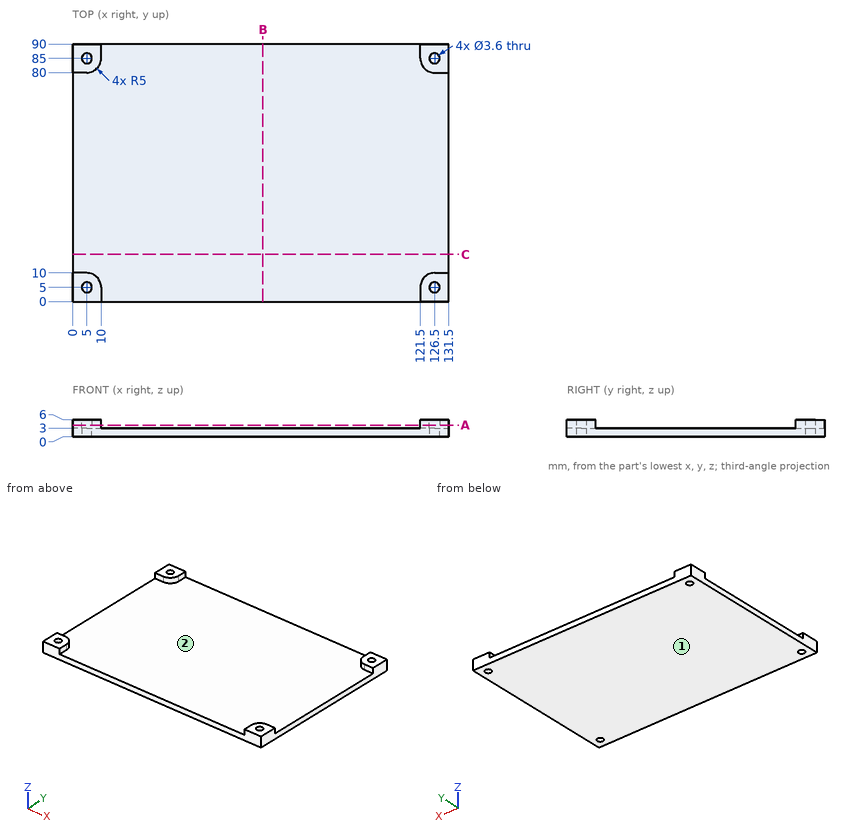
Answer from the drawing. Dimensions are ordinates in mm from the lowest x, y and z of the part. Coordinates: 2 decimals unless noted, no trailing zeros. Loops run counter-clockwise (first coordinate to the right, second up) from the corner with the lowest first, then second, coordinate; pieces in that order, holes last. Notation, with made-up numbers: (9.5, 62) -> (55.5, 62) arc R11 ccw to (55.5, 80) -> close; hole circle Ø7 at (41.5, 7). An arc over 180 degrees is marked (long way). Return JSON: item names as keys, results as strings.
Item 1: A flat-ended cylindrical pin translates along its axis: P1, Ø2.5, axis at x = 128, z = 4.5, coming from the -Y side. Find the tip coordinate at first contact, or state that the pin passes through.
Answers:
{"P1": "stops at y = 0"}
Item 2: For a pull along Z with two mould halves and no side action, classify the marked faces 1 and 2 as +Z half, -Z half, draft (parallel to the pull), parting line (faces both ways), or undercut.
Answers:
{"face 1": "-Z half", "face 2": "+Z half"}
Item 3: Find the intervals of material crossed by probe 1 along Y at (x, z) = (126.5, 4.4); probe 2 along X at (y, z) = (5, 2.4); probe 3 along Y at (x, z) = (5, 1.45), in increasing order.
Answers:
{"probe 1": "y = 0 to 3.2, 6.8 to 10, 80 to 83.2, 86.8 to 90", "probe 2": "x = 0 to 3.2, 6.8 to 124.7, 128.3 to 131.5", "probe 3": "y = 0 to 3.2, 6.8 to 83.2, 86.8 to 90"}
Item 4: Find section C-C (y = 16.5). Determine the outline of the cut face in (x, z).
Answers:
{"outline": "(0, 0) -> (131.5, 0) -> (131.5, 3) -> (0, 3) -> close"}
Item 5: Find section B-B (x = 66.5). Determine the outline of the cut face in (y, z).
Answers:
{"outline": "(0, 0) -> (90, 0) -> (90, 3) -> (0, 3) -> close"}
Item 6: Find section A-A (z = 4.05). Determine the outline of the cut face in (x, y), plus the area to 3 significant figures.
Answers:
{"outline": "(0, 0) -> (10, 0) -> (10, 5) arc R5 ccw to (5, 10) -> (0, 10) -> close; (0, 80) -> (5, 80) arc R5 ccw to (10, 85) -> (10, 90) -> (0, 90) -> close; (121.5, 0) -> (131.5, 0) -> (131.5, 10) -> (126.5, 10) arc R5 ccw to (121.5, 5) -> close; (121.5, 85) arc R5 ccw to (126.5, 80) -> (131.5, 80) -> (131.5, 90) -> (121.5, 90) -> close; hole circle Ø3.6 at (5, 5); hole circle Ø3.6 at (5, 85); hole circle Ø3.6 at (126.5, 5); hole circle Ø3.6 at (126.5, 85)", "area": "338 mm2"}
